Source: CAD feature listing. Evaluate the final solid. Frame: model axes, mm. A direction names the side the tool comes from. Give positions to 0.01 mm unless a question says otherwise; leave off trailing zeros. Order: outer loops, then holes, each group sorted by start corner. A loop starts at its lowest first (then second) coordinate and runs counter-clockwise, first axis right, second up.
1) Section C-C, the plane z = 0.5. Return loops of the section in (x, y) (3 decimals), plus the area to 3 significant figures.
2) First-contact query: P1, Ø3.5, axis at x = -8, y = 0, coming from the -Z side; P2, Ø4, axis at x = 3, z = -7.5, coming from the +Y side; P3, Ø6, axis at y = 2, z = -10.5, coming from the -X side. Flat tips, straight axial feed; report the tip coordinate or a pass-through.
3) Section D-D, the plane x = 8. Return loops of the section in (y, z) (3 decimals).
4) Section B-B, the plane y = -0.75. Return loops of the section in (x, z), plus the area to 3 significant figures.
5) Access query for faces 1 (the face through (0, 0, 0)), 2 (the face through (6.576, 0.063, 0.986)). Directions: +Z, -Z, +X, -X, +Y, -Y. A direction counts if a zero-diameter tool reaches every point of the face in a straight line with its end or side. Return the directions, or none.
6) Material intervals for line 1 (Y direction, x = 0, z = 0.6) (3 decimals); line 2 (Y direction, x = 0, z = -3.75); line 3 (Z direction, x = 3.25, y = 8.5), sorted ascending.
7) Draft query along X for faces 3 (the face through (-9.424, 0.063, 0.986)), 4 (the face through (-1.08, -4.88, -5.92)), 5 (the face through (5, -2, 0)), 6 (the face through (-0.186, -6.587, 0.986)). Return one class per face: released by +X, released by -X, zero draft, split by the parting line, or undercut.
8) Section A-A, the plane x = 0. Return loops of the section in (y, z) (3 decimals).
```python
from build123d import *

# Parameters (mm, degrees)
SKETCH1_R           = 11
SKETCH1_R_2         = 1.425
BOSS_EXTRUDE1_DEPTH = 2
SKETCH1_4_R         = 5
SKETCH1_4_R_2       = 1.5
BOSS_EXTRUDE2_DEPTH = 12


with BuildPart() as part:
    # Sketch1 → Boss-Extrude1 (new body)
    with BuildSketch(Plane.XY):
        Circle(SKETCH1_R)
        with Locations((0, 8)):
            Circle(SKETCH1_R_2, mode=Mode.SUBTRACT)
        with Locations((8, 0)):
            Circle(SKETCH1_R_2, mode=Mode.SUBTRACT)
        with Locations((0, -8)):
            Circle(SKETCH1_R_2, mode=Mode.SUBTRACT)
        with Locations((-8, 0)):
            Circle(SKETCH1_R_2, mode=Mode.SUBTRACT)
    extrude(amount=BOSS_EXTRUDE1_DEPTH)

    # Sketch1<4> → Boss-Extrude2 (add)
    with BuildSketch(Plane.XY):
        Circle(SKETCH1_4_R)
        Circle(SKETCH1_4_R_2, mode=Mode.SUBTRACT)
    extrude(amount=-BOSS_EXTRUDE2_DEPTH)


solid = part.part
```
From the geometry:
1. outline: circle Ø22 at (0, 0); hole circle Ø2.85 at (-8, 0); hole circle Ø2.85 at (0, -8); hole circle Ø2.85 at (0, 8); hole circle Ø2.85 at (8, 0)
1. area: 355 mm2
2. P1: stops at z = 0
2. P2: stops at y = 4.9
2. P3: stops at x = -5
3. outline: (-7.55, 0) - (-1.425, 0) - (-1.425, 2) - (-7.55, 2) - close; (1.425, 0) - (7.55, 0) - (7.55, 2) - (1.425, 2) - close
4. outline: (-10.97, 0) - (-9.21, 0) - (-9.21, 2) - (-10.97, 2) - close; (-6.79, 0) - (-4.94, 0) - (-4.94, -12) - (-1.3, -12) - (-1.3, 0) - (1.3, 0) - (1.3, -12) - (4.94, -12) - (4.94, 0) - (6.79, 0) - (6.79, 2) - (-6.79, 2) - close; (9.21, 0) - (10.97, 0) - (10.97, 2) - (9.21, 2) - close
4. area: 122 mm2
5. face 1: -Z
5. face 2: +Z, -Z
6. line 1: y = -11 to -9.425, -6.575 to 6.575, 9.425 to 11
6. line 2: y = -5 to -1.5, 1.5 to 5
6. line 3: z = 0 to 2
7. face 3: undercut
7. face 4: split by the parting line
7. face 5: zero draft
7. face 6: undercut
8. outline: (-11, 0) - (-9.425, 0) - (-9.425, 2) - (-11, 2) - close; (-6.575, 0) - (-5, 0) - (-5, -12) - (-1.5, -12) - (-1.5, 0) - (1.5, 0) - (1.5, -12) - (5, -12) - (5, 0) - (6.575, 0) - (6.575, 2) - (-6.575, 2) - close; (9.425, 0) - (11, 0) - (11, 2) - (9.425, 2) - close
